Part print with two shaded views. Sizes in mm from the minimum x, y, z corner. A direction names the side the tool comes from. Coordinates: 2 decimals unless noted, no trailing zeros. Loops run counter-clockwise (first coordinate to the right, second up) from the corner with the lowest first, then second, coordinate; pieces in that order, holes last. Notation, with made-up numbers: M 41.5,-2 L 47.5,-2 A21 cw 47.5,15 Z; hole C 59,13.5 d2. An arc over 180 degrees is marked long. Write item = value, one per line. Start each with the question number.
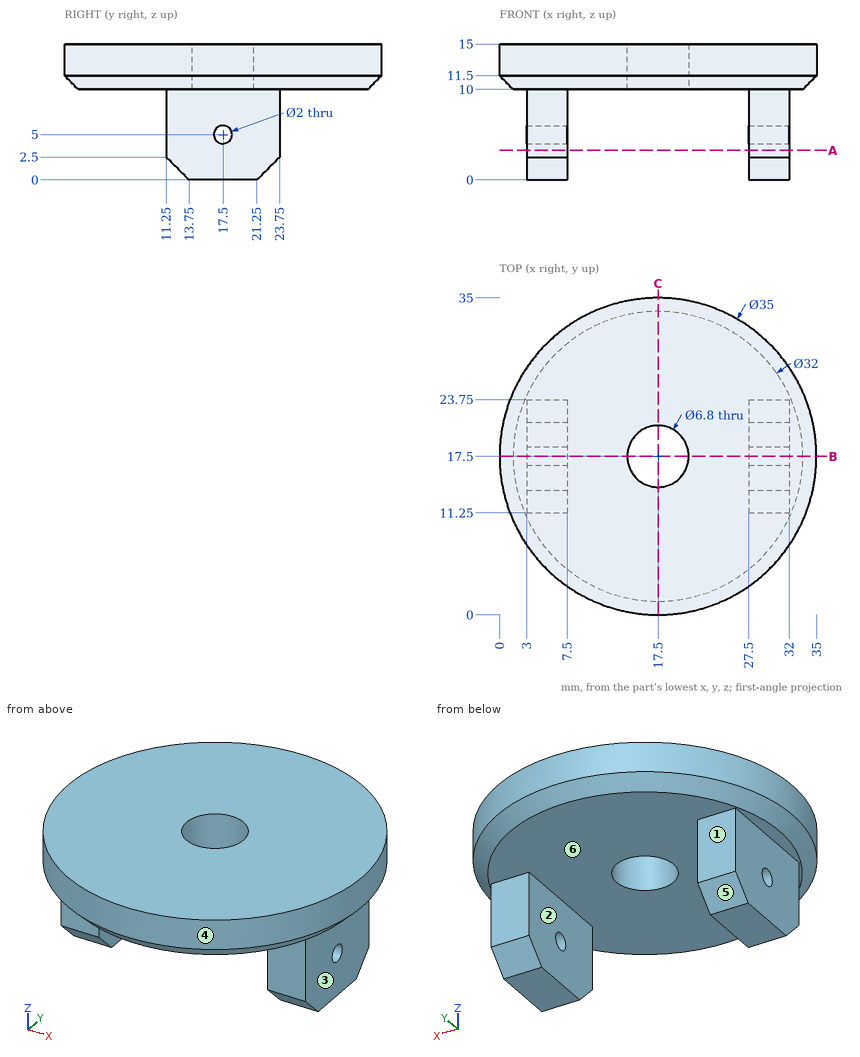
Item 1: Pull direction X, two halves, no side cores. Call the marked faces 4, 5 and 6: +X half, -X half, draft (parallel to the pull), parting line (faces both ways), or undercut.
Item 2: 3-axis set-ups, long thin cutter, end or side, ignore diameter. For the marked faces 1, 2 and 3: which of +Z, -Z, +X, -X, +Y, -Y reach the whole face in a straight line?
Item 3: Cut at C-C (x = 17.5). Give the cut face in (y, z), plus the area to 3 significant figures.
Item 4: Cut at A-A (z = 3.25). Give the cut face in (x, y), plus the area to 4 significant figures.
Item 5: Cut at B-B (y = 17.5). Give the cut face in (x, z), plus the area to 3 significant figures.
Item 6: Pin check, flat tips, straight feed: pin 1 Ø1.8 at (y, z) = (17.5, 5) entering from -X; pin 2 Ø8 at (x, y) = (9.5, 8.5) entering from -Z; pin 3 Ø5 at (y, z) = (16, 3.5) entering from +X; pin 4 Ø1.5 at (x, z) = (28, 7) entering from +Y. Stop position of each tip, or through.
Item 7: Probe L1, parallel to Y at x = 17.5, z = 12.2; L2, parallel to X at y = 22.5, z = 2.75; L3, parallel to Y at x = 4.5, z = 8.5. List the from-to ranges inside material, lowest first.
Reported:
q1.face_4 = parting line
q1.face_5 = draft
q1.face_6 = undercut
q2.face_1 = -Z, +X, -X, +Y
q2.face_2 = -Z, +Y, -Y
q2.face_3 = -Z, +X, +Y, -Y
q3.outline = M 0,11.5 L 1.5,10 L 14.1,10 L 14.1,15 L 0,15 Z; M 20.9,10 L 33.5,10 L 35,11.5 L 35,15 L 20.9,15 Z
q3.area = 139 mm^2
q4.outline = M 3,11.25 L 7.5,11.25 L 7.5,23.75 L 3,23.75 Z; M 27.5,11.25 L 32,11.25 L 32,23.75 L 27.5,23.75 Z
q4.area = 112.5 mm^2
q5.outline = M 0,11.5 L 1.5,10 L 3,10 L 3,6 L 7.5,6 L 7.5,10 L 14.1,10 L 14.1,15 L 0,15 Z; M 3,0 L 7.5,0 L 7.5,4 L 3,4 Z; M 20.9,10 L 27.5,10 L 27.5,6 L 32,6 L 32,10 L 33.5,10 L 35,11.5 L 35,15 L 20.9,15 Z; M 27.5,0 L 32,0 L 32,4 L 27.5,4 Z
q5.area = 211 mm^2
q6.pin_1 = through
q6.pin_2 = 1.79
q6.pin_3 = 32
q6.pin_4 = 23.75
q7.L1 = 0 to 14.1, 20.9 to 35
q7.L2 = 3 to 7.5, 27.5 to 32
q7.L3 = 11.25 to 23.75
